Work out the finished part from the listing and answer in its coordinate system (mm). Give positions to 0.01 mm unless a question says otherwise; leave off trailing zeros. Loops run counter-clockwise (first coordinate to the right, second up) from the corner with the lowest first, then second, coordinate; pieces in that order, holes last. Notation, with made-up numbers: M 33,-8.5 L 59,-8.5 A15 cw 59,9.5 Z; hole C 6.5,-39 d7. An arc over 180 degrees is marked long. Answer in a Markdown table with one row per item. Add a question column.
from build123d import *

# Parameters (mm, degrees)
SKETCH020_W     = 57
SKETCH020_H     = 76
SKETCH020_R     = 3.5
SKETCH020_R_2   = 1.3
SKETCH020_R_3   = 2.0625
SKETCH020_W_2   = 14.1
SKETCH020_H_2   = 14.1
PAD005_DEPTH    = 3
SKETCH022_W     = 15
SKETCH022_H     = 13
POCKET013_DEPTH = 2
FILLET005_R     = 1
SKETCH027_R     = 2.5
POCKET017_DEPTH = 1


with BuildPart() as part:
    # Sketch020 → Pad005 (new body)
    with BuildSketch(Plane.XY):
        with Locations((28.5, 38)):
            Rectangle(SKETCH020_W, SKETCH020_H)
        with Locations((47.5, 66.5)):
            Circle(SKETCH020_R, mode=Mode.SUBTRACT)
        with Locations((9.5, 57)):
            Circle(SKETCH020_R_2, mode=Mode.SUBTRACT)
        with Locations((9.5, 19)):
            Circle(SKETCH020_R_2, mode=Mode.SUBTRACT)
        with Locations((47.5, 19)):
            Circle(SKETCH020_R_2, mode=Mode.SUBTRACT)
        with Locations((47.5, 57)):
            Circle(SKETCH020_R_2, mode=Mode.SUBTRACT)
        with Locations((9.5, 38)):
            Circle(SKETCH020_R_2, mode=Mode.SUBTRACT)
        with Locations((47.5, 38)):
            Circle(SKETCH020_R_2, mode=Mode.SUBTRACT)
        with Locations((28.5, 66.5)):
            Circle(SKETCH020_R_3, mode=Mode.SUBTRACT)
        with Locations((9.5, 9.5)):
            Rectangle(SKETCH020_W_2, SKETCH020_H_2, mode=Mode.SUBTRACT)
        with Locations((9.5, 28.5)):
            Rectangle(SKETCH020_W_2, SKETCH020_H_2, mode=Mode.SUBTRACT)
        with Locations((9.5, 47.5)):
            Rectangle(SKETCH020_W_2, SKETCH020_H_2, mode=Mode.SUBTRACT)
        with Locations((9.5, 66.5)):
            Rectangle(SKETCH020_W_2, SKETCH020_H_2, mode=Mode.SUBTRACT)
        with Locations((28.5, 28.5)):
            Rectangle(SKETCH020_W_2, SKETCH020_H_2, mode=Mode.SUBTRACT)
        with Locations((47.5, 28.5)):
            Rectangle(SKETCH020_W_2, SKETCH020_H_2, mode=Mode.SUBTRACT)
        with Locations((28.5, 9.5)):
            Rectangle(SKETCH020_W_2, SKETCH020_H_2, mode=Mode.SUBTRACT)
        with Locations((47.5, 9.5)):
            Rectangle(SKETCH020_W_2, SKETCH020_H_2, mode=Mode.SUBTRACT)
        with BuildLine():
            ThreePointArc((21.75, 74.5), (21, 75.25), (20.25, 74.5))
            Line((20.25, 74.5), (20.25, 58.5))
            ThreePointArc((20.25, 58.5), (21, 57.75), (21.75, 58.5))
            Line((21.75, 74.5), (21.75, 58.5))
        make_face(mode=Mode.SUBTRACT)
        with BuildLine():
            ThreePointArc((36.75, 74.5), (36, 75.25), (35.25, 74.5))
            Line((35.25, 74.5), (35.25, 58.5))
            ThreePointArc((35.25, 58.5), (36, 57.75), (36.75, 58.5))
            Line((36.75, 58.5), (36.75, 74.5))
        make_face(mode=Mode.SUBTRACT)
    extrude(amount=PAD005_DEPTH)

    # Sketch022 → Pocket013 (cut)
    with BuildSketch(Plane(origin=(0, 0, 0), x_dir=(1, 0, 0), z_dir=(0, 0, -1))):
        with Locations((47.5, -66.5)):
            Rectangle(SKETCH022_W, SKETCH022_H)
    extrude(amount=-POCKET013_DEPTH, mode=Mode.SUBTRACT)

    # Fillet005
    fillet005_edges = [part.edges().sort_by_distance(p)[0] for p in [
        (0, 0, 1.5),
        (57, 0, 1.5),
        (57, 76, 1.5),
        (0, 76, 1.5),
    ]]
    fillet(fillet005_edges, radius=FILLET005_R)

    # Sketch027 (on Face5 of Fillet005) → Pocket017 (cut)
    with BuildSketch(Plane.XY.offset(3)):
        with Locations((9.5, 57)):
            Circle(SKETCH027_R)
        with Locations((9.5, 38)):
            Circle(SKETCH027_R)
        with Locations((47.5, 57)):
            Circle(SKETCH027_R)
        with Locations((47.5, 38)):
            Circle(SKETCH027_R)
        with Locations((47.5, 19)):
            Circle(SKETCH027_R)
        with Locations((9.5, 19)):
            Circle(SKETCH027_R)
    extrude(amount=-POCKET017_DEPTH, mode=Mode.SUBTRACT)


with BuildPart() as part_1:
    # Body004 placement: moved
    add(part.part.moved(Location((6, 6, 11))))


solid = part_1.part
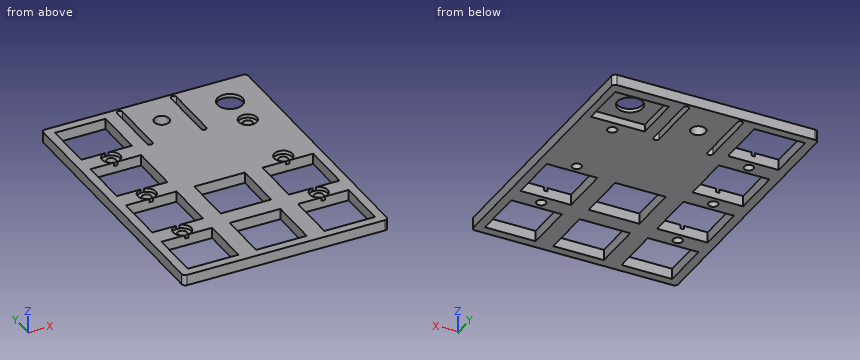
(1) Section B-B, the plane y = 72.5 is taken. Determine the outline of the cut face in (x, z).
(2) Consider line 1 along Y through (x, z) = (37.5, 13.3); line 2 along Y through (x, z) = (34.5, 11.7); line 3 along X through (y, z) = (63, 12.35). Determine where each line is inside the solid, lowest interval first. Write a range as from..to.
(3) Section C-C, the plane y = 15.5 is taken. Determine the outline of the cut face in (x, z).
(4) Section A-A, the plane x = 40 is taken. Determine the outline of the cut face in (y, z).
(5) Each of these flat-tipped pins is pushed along its axis until it touches: P1, Ø2.5, axis at x = 54.5, y = 63.5, coming from the +Z side; P2, Ø1.6, axis at x = 15.5, y = 63, coming from the +Z side. Where does it stop, or does it pass through?
(6) Section D-D, the plane x = 58 is taken. Determine the outline of the cut face in (y, z), and give its area (3 significant figures).
Numbers:
| question | item | result |
|---|---|---|
| 1 | outline | M 6,11 L 8.45,11 L 8.45,14 L 6,14 Z; M 22.55,11 L 26.25,11 L 26.25,14 L 22.55,14 Z; M 27.75,11 L 32.44,11 L 32.44,14 L 27.75,14 Z; M 36.56,11 L 41.25,11 L 41.25,14 L 36.56,14 Z; M 42.75,11 L 46,11 L 46,13 L 50,13 L 50,14 L 42.75,14 Z; M 57,13 L 61,13 L 61,11 L 63,11 L 63,14 L 57,14 Z |
| 2 | line 1 | y = 6..8.45, 22.55..27.45, 41.55..82 |
| 2 | line 2 | y = 6..8.45, 22.55..27.45, 41.55..70.44, 74.56..82 |
| 2 | line 3 | x = 6..14.2, 16.8..52.2, 54.8..63 |
| 3 | outline | M 6,11 L 8.45,11 L 8.45,14 L 6,14 Z; M 22.55,11 L 27.45,11 L 27.45,14 L 22.55,14 Z; M 41.55,11 L 46.45,11 L 46.45,14 L 41.55,14 Z; M 60.55,11 L 63,11 L 63,14 L 60.55,14 Z |
| 4 | outline | M 6,11 L 8.45,11 L 8.45,14 L 6,14 Z; M 22.55,11 L 27.45,11 L 27.45,14 L 22.55,14 Z; M 41.55,11 L 82,11 L 82,14 L 41.55,14 Z |
| 5 | P1 | stops at z = 13 |
| 5 | P2 | passes through |
| 6 | outline | M 6,11 L 8.45,11 L 8.45,14 L 6,14 Z; M 22.55,11 L 27.45,11 L 27.45,14 L 22.55,14 Z; M 41.55,11 L 66,11 L 66,13 L 79,13 L 79,11 L 82,11 L 82,14 L 41.55,14 Z |
| 6 | area | 117 mm² |
